The listing builds one solid part. Answer for the finished solid, in the listing's coordinates (mm). A direction names the side the tool comes from. Give positions to 0.01 mm unless a question says otherwise; leave off trailing zeros. Loops run counter-clockwise (first coordinate to the right, second up) from the corner with the lowest first, then second, coordinate; pieces in that order, holes last. Notation, with made-up numbers: M 42,-32 L 54,-32 A25 cw 54,-9 Z; hole C 52.25,48.5 d3. An arc over 180 degrees is marked long. One line per item, written item: value. Start each with the question number.
Q1. The mould has two halves that part along Y. Classify faces 3 (the flat face through (-32, 0, 5)), 4 (the flat face through (-36.71, 4.696, 17.835)), 5 (the cylindrical face through (-42.233, 6.812, 5.452)): +Y half, -Y half, draft (parallel to the pull), parting line (faces both ways), or undercut.
Q2. Consider L1, parallel to X at y = 5.75, z = 7.5; L2, parallel to Z at x = -36.75, y = 3.25; L3, parallel to X at y = 0.75, z = -3. Determine where each line is inside the solid, lowest interval first.
Q3. For faces 1 (the flat face through (-41.03, 5.09, -5.68)), 2 (the flat face through (-33.49, 4.7, -7.36)), determine the directions among +Z, -Z, +X, -X, +Y, -Y from which every point of the face is accessible in a straight line to the end or side of a thin tool.
Q4. Flat-ended cylindrical pins translate along their axes: pin 1 (1 mm diameter, centred on y = 1.5, z = 1, fed in from -X); pin 2 (6 mm diameter, centred on x = -43, z = -1.5, fed in from +Y); pin 3 (3 mm diameter, centred on x = -32, y = 5.5, fed in from +Z). Find the tip coordinate at first contact, or state that the pin passes through.
Q5. A cutting plane is placed at A-A, the plane x = -35.5. Determine the outline of the cut face in (y, z) (3 decimals).
from build123d import *

# Parameters (mm, degrees)
BOSS_EXTRUDE1_DEPTH = 9.525
SKETCH3_R           = 2.032
CUT_EXTRUDE1_DEPTH  = 2.7
SKETCH4_R           = 1.000000032
CUT_EXTRUDE2_DEPTH  = 51.984772229
FILLET2_SIZE        = 6.096


with BuildPart() as part:
    # Sketch1 → Boss-Extrude1 (new body)
    with BuildSketch(Plane(origin=(0, 0, 0), x_dir=(1, 0, 0), z_dir=(0, 1, 0))):
        Polygon((-27.422743224, -19.119856123), (-46.29298428, -16.509012872), (-42.811859946, 8.651308536), (-23.941618889, 6.040465285), align=None)
    extrude(amount=BOSS_EXTRUDE1_DEPTH)

    # Sketch3 → Cut-Extrude1 (cut)
    with BuildSketch(Plane(origin=(0.316670388, 0, -2.684144047), x_dir=(-0.9905638349724136, 0, -0.13705213914691383), z_dir=(0.13705213914691383, 0, -0.9905638349724136))):
        with Locations((40.495544979, 5.969)):
            Circle(SKETCH3_R)
    extrude(amount=-CUT_EXTRUDE1_DEPTH, mode=Mode.SUBTRACT)

    # Sketch4 → Cut-Extrude2 (cut, through all)
    with BuildSketch(Plane(origin=(0.000303759, 0, -0.00219546), x_dir=(-0.9905638349724136, 0, -0.13705213914691383), z_dir=(0.1370521391469138, 0, -0.9905638349724135))):
        with Locations((40.549730429, 5.969)):
            Circle(SKETCH4_R)
    extrude(amount=-CUT_EXTRUDE2_DEPTH, mode=Mode.SUBTRACT)

    # Fillet2
    # a fillet whose section is not a circle: 6.096 mm, written as the material it takes off along each edge
    with BuildSketch(Plane(origin=(-48.38165888, 0, 31.605205717), x_dir=(0.9905638349724136, 0, 0.13705213914691353), z_dir=(0.13705213914691353, 0, -0.9905638349724136))) as fillet2_piece_1:
        with BuildLine():
            add(Edge.make_bspline([(FILLET2_SIZE, 0), (FILLET2_SIZE * 0.831801948466, 0), (FILLET2_SIZE * 0.663603896932, 0), (FILLET2_SIZE * 0.292893218813, -FILLET2_SIZE * 0.0716919198361), (FILLET2_SIZE * 0.0716919198361, -FILLET2_SIZE * 0.292893218813), (0, -FILLET2_SIZE * 0.663603896932), (0, -FILLET2_SIZE * 0.831801948466), (0, -FILLET2_SIZE)], knots=[0, 0, 0, 0, 0, 0, 0.5, 0.5, 1, 1, 1, 1, 1, 1], degree=5))
            Line((0, -FILLET2_SIZE), (0, 0))
            Line((0, 0), (FILLET2_SIZE, 0))
        make_face()
    extrude(amount=55.88, mode=Mode.SUBTRACT)
    with BuildSketch(Plane(origin=(-48.38165888, 9.525, 31.605205717), x_dir=(0.9905638349724136, 0, 0.13705213914691353), z_dir=(0.13705213914691353, 0, -0.9905638349724136))) as fillet2_piece_2:
        with BuildLine():
            add(Edge.make_bspline([(FILLET2_SIZE, 0), (FILLET2_SIZE * 0.831801948466, 0), (FILLET2_SIZE * 0.663603896932, 0), (FILLET2_SIZE * 0.292893218813, FILLET2_SIZE * 0.0716919198361), (FILLET2_SIZE * 0.0716919198361, FILLET2_SIZE * 0.292893218813), (0, FILLET2_SIZE * 0.663603896932), (0, FILLET2_SIZE * 0.831801948466), (0, FILLET2_SIZE)], knots=[0, 0, 0, 0, 0, 0, 0.5, 0.5, 1, 1, 1, 1, 1, 1], degree=5))
            Line((0, FILLET2_SIZE), (0, 0))
            Line((0, 0), (FILLET2_SIZE, 0))
        make_face()
    extrude(amount=55.88, mode=Mode.SUBTRACT)


solid = part.part
Answer block:
1. face 3: -Y half
1. face 4: draft
1. face 5: undercut
2. L1: -44.89 to -42.96, -40.99 to -25.82
2. L2: -7.81 to 17.83
2. L3: -41.46 to -24.36
3. face 1: none
3. face 2: -Z, +X, +Y, -Y
4. pin 1: x = -43.33
4. pin 2: y = 9.37
4. pin 3: z = 18.69
5. outline: M 0,-7.64 L 9.525,-7.64 L 9.525,18.002 L 0,18.002 Z
